Model file for the job. Use its own axes, mm. Face numbers are marked on the shaded views. A direction names the side the tool comes from. Round coordinates to 2 decimals unless told otherwise and drop trailing zeros. Order: outer loops, then holes, each group sorted by start corner. A loop starts at its lowest first (then second) coordinate and runs counter-clockwise, first axis right, second up. Notation, with made-up numbers: (38.5, 31.5) -> (47.5, 31.5) arc R24 cw to (47.5, 64.5) -> close; hole circle Ø11 at (-32.5, 51). An arc over 180 degrees is marked (long way). Put each result on its own line as item: value. Start each with the question number.
Q1. 3-axis set-ups, long thin cutter, end or side, ignore diameter. For the marked faces 1 and 2: which of +Z, -Z, +X, -X, +Y, -Y reach the whole face in a straight line?
Q2. Flat gauge pins, fed straight in: P1, Ø6, axis at x = -8.2, z = -172.5, coming from the -Y side; P2, Ø1.5, axis at y = 49.5, z = -150, coming from the -X side; P3, Ø0.8, axis at x = -0.5, z = -95.5, coming from the -Y side; P4, Ø7, axis at x = -8.5, z = -10, coming from the +Y side. Where does each tip first touch, or does it go through?
Q3. Probe L1, parallel to Z at x = -8.2, y = -61.1; L2, parallel to Y at x = -0.5, z = -30; L3, parallel to X at y = -51, z = -162.5. List the from-to ranges inside material, lowest first.
Q4. Cut at B-B, the plane y = 52. List the corners of the cut face in (x, z).
Q5. Cut at A-A, the plane z = -137. List the corners of the cut face in (x, y), and give its area (3 significant figures).
from build123d import *

# Parameters (mm, degrees)
BASE_FLANGE1_START        = -0.7
BASE_FLANGE1_OUTLINE_W    = 150
BASE_FLANGE1_OUTLINE_H    = 40
BASE_FLANGE1_OUTLINE_W_2  = 125
BASE_FLANGE1_DEPTH        = 0.7
CUT_EXTRUDE1_DEPTH        = 10
EDGE_FLANGE3_DEPTH        = 15
EDGE_FLANGE2_DEPTH        = 15
F_6_CLEARANCE_HOLE1_D     = 3.7973
F_6_CLEARANCE_HOLE1_DEPTH = 10
F_6_CLEARANCE_HOLE1_TIP   = 1.140824014
CUT_EXTRUDE2_DEPTH        = 10
BREAK_CORNER1_START       = -61.4366
BREAK_CORNER1_DEPTH       = 0.7
BREAK_CORNER1_START_2     = -0.7
BREAK_CORNER1_2_DEPTH     = 0.7
FILLET1_R                 = 2.5


# Read off the part's stored shape, not the designer's step: Base-Flange1, Break-Corner1
# Sheet-metal steps are written as plain solids
with BuildPart() as part:
    # Base-Flange1 outline → Base-Flange1 (new body)
    with BuildSketch(Plane(origin=(0, 0, 0), x_dir=(0, 0, -1), z_dir=(1, 0, 0)).offset(BASE_FLANGE1_START)):
        Polygon((180, 110), (0, 110), (0, -60), (15, -60), (15, -40), (100, -40), (100, -60), (180, -60), align=None)
        with Locations((90, 20)):
            Rectangle(BASE_FLANGE1_OUTLINE_W, BASE_FLANGE1_OUTLINE_H, mode=Mode.SUBTRACT)
        with Locations((102.5, 75)):
            Rectangle(BASE_FLANGE1_OUTLINE_W_2, BASE_FLANGE1_OUTLINE_H, mode=Mode.SUBTRACT)
    extrude(amount=BASE_FLANGE1_DEPTH)

    # Sketch4 → Cut-Extrude1 (cut)
    with BuildSketch(Plane(origin=(0, 0, 0), x_dir=(0, 0, -1), z_dir=(1, 0, 0))):
        with BuildLine():
            Line((25.3, -15), (25.3, -35))
            ThreePointArc((25.3, -35), (24.8, -35.5), (24.3, -35))
            Line((24.3, -35), (24.3, -15))
            ThreePointArc((24.3, -15), (24.8, -14.5), (25.3, -15))
        make_face()
    extrude(amount=-CUT_EXTRUDE1_DEPTH, mode=Mode.SUBTRACT)

    # Edge-Flange3 section (across the edge) → Edge-Flange3 (add)
    with BuildSketch(Plane(origin=(-0.7, -60.7366, -180), x_dir=(0, 1, 0), z_dir=(0, 0, 1))):
        with BuildLine():
            Line((-0.7, 0.7366), (-0.7, 15))
            Line((-0.7, 15), (0, 15))
            Line((0, 15), (0, 0.7366))
            ThreePointArc((0, 0.7366), (0.215745145, 0.215745145), (0.7366, 0))
            Line((0.7366, 0), (0.7366, -0.7))
            ThreePointArc((0.7366, -0.7), (-0.279229602, -0.279229602), (-0.7, 0.7366))
        make_face()
    extrude(amount=EDGE_FLANGE3_DEPTH)

    # Edge-Flange2 section (across the edge) → Edge-Flange2 (add)
    with BuildSketch(Plane(origin=(-0.7, -60.7366, -15), x_dir=(0, 1, 0), z_dir=(0, 0, 1))):
        with BuildLine():
            Line((-0.7, 0.7366), (-0.7, 15))
            Line((-0.7, 15), (0, 15))
            Line((0, 15), (0, 0.7366))
            ThreePointArc((0, 0.7366), (0.215745145, 0.215745145), (0.7366, 0))
            Line((0.7366, 0), (0.7366, -0.7))
            ThreePointArc((0.7366, -0.7), (-0.279229602, -0.279229602), (-0.7, 0.7366))
        make_face()
    extrude(amount=EDGE_FLANGE2_DEPTH)

    # #6 Clearance Hole1
    with Locations(Plane(origin=(0, -60.7366, 0), x_dir=(1, 0, 0), z_dir=(0, 1, 0))):
        with Locations((-8.2, 7.5), (-8.2, 172.5)):
            Hole(F_6_CLEARANCE_HOLE1_D / 2, depth=F_6_CLEARANCE_HOLE1_DEPTH)
            with Locations((0, 0, -(F_6_CLEARANCE_HOLE1_DEPTH + F_6_CLEARANCE_HOLE1_TIP / 2))):  # 118° drill point
                Cone(0, F_6_CLEARANCE_HOLE1_D / 2, F_6_CLEARANCE_HOLE1_TIP, mode=Mode.SUBTRACT)

    # Sketch13 → Cut-Extrude2 (cut)
    with BuildSketch(Plane(origin=(0, 0, 0), x_dir=(0, 0, -1), z_dir=(1, 0, 0))):
        with BuildLine():
            Line((9.2, 105), (9.2, 95))
            ThreePointArc((9.2, 95), (7.5, 93.3), (5.8, 95))
            Line((5.8, 95), (5.8, 105))
            ThreePointArc((5.8, 105), (7.5, 106.7), (9.2, 105))
        make_face()
        with BuildLine():
            Line((174.2, 105), (174.2, 95))
            ThreePointArc((174.2, 95), (172.5, 93.3), (170.8, 95))
            Line((170.8, 95), (170.8, 105))
            ThreePointArc((170.8, 105), (172.5, 106.7), (174.2, 105))
        make_face()
        with BuildLine():
            Line((9.2, 60), (9.2, 50))
            ThreePointArc((9.2, 50), (7.5, 48.3), (5.8, 50))
            Line((5.8, 50), (5.8, 60))
            ThreePointArc((5.8, 60), (7.5, 61.7), (9.2, 60))
        make_face()
        with BuildLine():
            Line((174.2, 60), (174.2, 50))
            ThreePointArc((174.2, 50), (172.5, 48.3), (170.8, 50))
            Line((170.8, 50), (170.8, 60))
            ThreePointArc((170.8, 60), (172.5, 61.7), (174.2, 60))
        make_face()
    extrude(amount=-CUT_EXTRUDE2_DEPTH, mode=Mode.SUBTRACT)

    # Break-Corner1 outline → Break-Corner1 (cut)
    with BuildSketch(Plane(origin=(0, 0, 0), x_dir=(1, 0, 0), z_dir=(0, 1, 0)).offset(BREAK_CORNER1_START)):
        with BuildLine():
            ThreePointArc((-13.2, 0), (-14.967766953, 0.732233047), (-15.7, 2.5))
            Line((-15.7, 2.5), (-15.7, 0))
            Line((-15.7, 0), (-13.2, 0))
        make_face()
        with BuildLine():
            ThreePointArc((-15.7, 12.5), (-14.967766953, 14.267766953), (-13.2, 15))
            Line((-13.2, 15), (-15.7, 15))
            Line((-15.7, 15), (-15.7, 12.5))
        make_face()
        with BuildLine():
            Line((-15.7, 180), (-15.7, 177.5))
            ThreePointArc((-15.7, 177.5), (-14.967766953, 179.267766953), (-13.2, 180))
            Line((-13.2, 180), (-15.7, 180))
        make_face()
        with BuildLine():
            ThreePointArc((-13.2, 165), (-14.967766953, 165.732233047), (-15.7, 167.5))
            Line((-15.7, 167.5), (-15.7, 165))
            Line((-15.7, 165), (-13.2, 165))
        make_face()
    extrude(amount=BREAK_CORNER1_DEPTH, mode=Mode.SUBTRACT)

    # Break-Corner1 2 outline → Break-Corner1 2 (cut)
    with BuildSketch(Plane.YZ.offset(BREAK_CORNER1_START_2)):
        with BuildLine():
            ThreePointArc((107.5, 0), (109.267766953, -0.732233047), (110, -2.5))
            Line((110, -2.5), (110, 0))
            Line((110, 0), (107.5, 0))
        make_face()
        with BuildLine():
            ThreePointArc((110, -177.5), (109.267766953, -179.267766953), (107.5, -180))
            Line((107.5, -180), (110, -180))
            Line((110, -180), (110, -177.5))
        make_face()
        with BuildLine():
            ThreePointArc((-60, -102.5), (-59.267766953, -100.732233047), (-57.5, -100))
            Line((-57.5, -100), (-60, -100))
            Line((-60, -100), (-60, -102.5))
        make_face()
    extrude(amount=BREAK_CORNER1_2_DEPTH, mode=Mode.SUBTRACT)

    # Fillet1
    fillet1_edges = [part.edges().sort_by_distance(p)[0] for p in [
        (-0.35, 55, -40),
        (-0.35, 95, -40),
        (-0.35, 95, -165),
        (-0.35, 55, -165),
        (-0.35, 40, -165),
        (-0.35, 0, -165),
        (-0.35, 0, -15),
        (-0.35, 40, -15),
    ]]
    fillet(fillet1_edges, radius=FILLET1_R)


solid = part.part
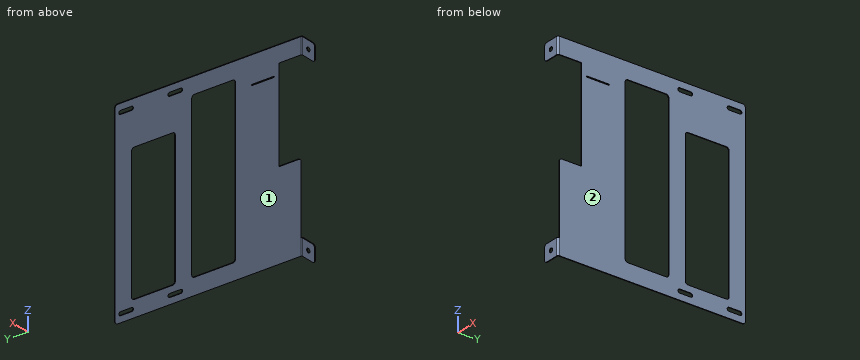
Ans:
1. face 1: +Z, -Z, -X, +Y
1. face 2: +Z, -Z, +X, +Y, -Y
2. P1: stops at y = -61.44
2. P2: stops at x = -0.7
2. P3: stops at y = -40
2. P4: stops at y = -60.74
3. L1: z = -180 to -174.4, -170.6 to -165, -15 to -9.4, -5.6 to 0
3. L2: y = -40 to 0, 40 to 110
3. L3: x = -0.7 to 0
4. outline: (-0.7, -180) -> (0, -180) -> (0, -174.2) -> (-0.7, -174.2) -> close; (-0.7, -170.8) -> (0, -170.8) -> (0, -9.2) -> (-0.7, -9.2) -> close; (-0.7, -5.8) -> (0, -5.8) -> (0, 0) -> (-0.7, 0) -> close
5. outline: (-0.7, -60) -> (0, -60) -> (0, 0) -> (-0.7, 0) -> close; (-0.7, 40) -> (0, 40) -> (0, 55) -> (-0.7, 55) -> close; (-0.7, 95) -> (0, 95) -> (0, 110) -> (-0.7, 110) -> close
5. area: 63.0 mm^2
